from build123d import *

# Parameters (mm, degrees)
SKETCH1_R           = 12.7
BOSS_EXTRUDE1_DEPTH = 609.6
SKETCH2_R           = 3.96875
BOSS_EXTRUDE2_DEPTH = 38.1


with BuildPart() as part:
    # Sketch1 → Boss-Extrude1 (new body)
    with BuildSketch(Plane(origin=(0, 0, 0), x_dir=(0, 0, -1), z_dir=(1, 0, 0))):
        with Locations(Location((0, 0, 0), (0, 0, 180))):
            Circle(SKETCH1_R)
    extrude(amount=BOSS_EXTRUDE1_DEPTH)

    # Sketch2 → Boss-Extrude2 (add, symmetric)
    with BuildSketch(Plane.XY):
        with Locations((7.62, 0)):
            Circle(SKETCH2_R)
        with Locations(Location((601.98, 0, 0), (0, 0, 180))):
            Circle(SKETCH2_R)
    extrude(amount=BOSS_EXTRUDE2_DEPTH, both=True)


solid = part.part
Can you work these out from the model? Positions are in its coordinate system, mm. Round coordinates to 2 decimals unless told otherwise and drop trailing zeros. Write each loop counter-clockwise with the first axis right and the second up, starting at its lowest first coordinate (ties: lowest second). Pieces come first, ordered by that corner, then holes. Notation, with made-up numbers: M 32.25,9.25 L 54.25,9.25 A27 ccw 54.25,33.25 Z; hole C 13,0.25 d1. An arc over 180 degrees is marked long. Use a Markdown table: item, result.
Item 1: If I drill on line 1 along X through (y, z) = (-2.25, 17); line 2 along Y through (x, z) = (583, 1); line 3 along Y through (x, z) = (448, 4), over which ranges is the centre line in solid material (lowest first)? Write a range as [from, to].
Found:
| item | result |
|---|---|
| line 1 | x = [4.35, 10.89], [598.71, 605.25] |
| line 2 | y = [-12.66, 12.66] |
| line 3 | y = [-12.05, 12.05] |
Item 2: For pin 1 Ø12 at (x, y) = (87, -8) entering from -Z; pin 2 Ø1 at (x, y) = (488, 9) entering from -Z; pin 3 Ø8 at (x, y) = (316, 3.5) entering from -Z, each with a flat end and sliding along its axis, tell me the tip position at first contact or that it passes through.
Found:
| item | result |
|---|---|
| pin 1 | stops at z = -12.54 |
| pin 2 | stops at z = -9.44 |
| pin 3 | stops at z = -12.7 |
Item 3: We'd pull the mould along X, two halves only. Please class faces 1 (the face through (0, 0, 0)), 2 (the face through (300.533, 11.267, 5.86)), 3 (the face through (609.6, 0, 0)): released by +X, released by -X, zero draft, split by the parting line, or undercut.
Found:
| item | result |
|---|---|
| face 1 | released by -X |
| face 2 | undercut |
| face 3 | released by +X |
Item 4: I want a section at C-C (x = 254). List the corners of the cut face in (y, z) for me, and give its area (3 significant figures).
Found:
| item | result |
|---|---|
| outline | C 0,0 d25.4 |
| area | 507 mm2 |
Item 5: I want a section at A-A (y = 0). List the corners of the cut face in (x, z) for me.
Found:
| item | result |
|---|---|
| outline | M 0,-12.7 L 3.65,-12.7 L 3.65,-38.1 L 11.59,-38.1 L 11.59,-12.7 L 598.01,-12.7 L 598.01,-38.1 L 605.95,-38.1 L 605.95,-12.7 L 609.6,-12.7 L 609.6,12.7 L 605.95,12.7 L 605.95,38.1 L 598.01,38.1 L 598.01,12.7 L 11.59,12.7 L 11.59,38.1 L 3.65,38.1 L 3.65,12.7 L 0,12.7 Z |
Item 6: I want a section at D-D (z = -4.5). List the corners of the cut face in (x, y) for me.
Found:
| item | result |
|---|---|
| outline | M 0,-11.88 L 609.6,-11.88 L 609.6,11.88 L 0,11.88 Z |
Item 7: I want a section at B-B (z = -29). List the corners of the cut face in (x, y) for me.
Found:
| item | result |
|---|---|
| outline | C 7.62,0 d7.94; C 601.98,0 d7.94 |
